Input: dimensioned drawing with shaded views. Units: mm. Origin: part minimum x, y, z. A direction names the side the tool comes from. Round coordinates to 2 decimals unless told otherwise and drop trailing zeros. Loops run counter-clockwise (first coordinate to the right, second up) from the corner with the lowest first, then second, coordinate; pieces in that order, holes last. Notation, with made-up numbers: (86.5, -4.5) - (133.5, -4.5) arc R23 cw to (133.5, 14.5) - close; hole circle Ø6 at (89.25, -23.75). An arc over 180 degrees is marked (long way). Answer as a JSON object with one key per item and string values. Group by question number.
Item 1: First-contact query: pin 1 (5 mm diameter, centred on x = 8.5, z = 10, fed in from -Y); pin 2 (10 mm diameter, centred on x = 17.5, z = 19, fed in from +Y); pin 3 (10 mm diameter, centred on y = 18.5, z = 9, fed in from +X). Flat tips, straight axial feed; report the tip coordinate or a pass-through.
Item 2: Section A-A (x = 12.5). Return the cut outline in (y, z).
Item 3: Reachability of the marked faces 1 and 2 from +Z, -Z, +X, -X, +Y, -Y: full face, straight path, thin tool, end or side. Return the list, or none.
Item 4: Line query: line 1 (X direction, y = 12.75, z = 9.5); line 2 (Y direction, x = 12, z = 6.5); line 3 (Y direction, x = 9.5, z = 43). Output: solid intervals per line, ascending.
Item 5: Section C-C (z = 47). Return the cut outline in (x, y).
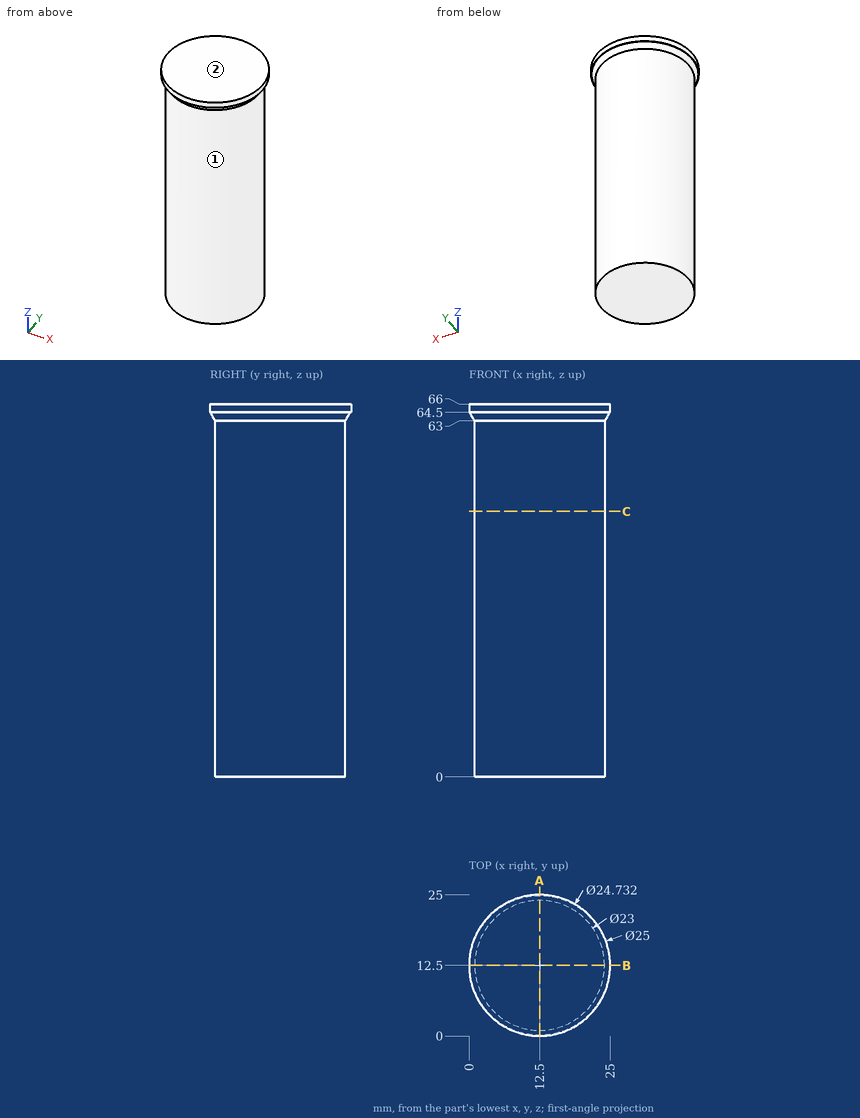
Values:
{
 "1": {"pin 1": "stops at y = 1.1", "pin 2": "stops at y = 24", "pin 3": "stops at x = 23.96"},
 "2": {"outline": "(0, 64.5) - (0.13, 64.5) - (1, 63) - (1, 0) - (24, 0) - (24, 63) - (24.87, 64.5) - (25, 64.5) - (25, 66) - (0, 66) - close"},
 "3": {"face 1": "-Z", "face 2": "+Z, +X, -X, +Y, -Y"},
 "4": {"line 1": "x = 1 to 24", "line 2": "y = 1.01 to 23.99", "line 3": "y = 1.4 to 23.6"},
 "5": {"outline": "circle Ø23 at (12.5, 12.5)"}
}
